Can you work these out from the model? Positions are in its coordinate system, mm. Face numbers are marked on the shaded views. A direction names the side the tool comes from. Give positions to 0.01 mm unless a question says otherwise; leave off trailing zeros. Loops run counter-clockwise (first coordinate to the right, second up) from the corner with the lowest first, then second, coordinate; pieces in that order, holes last. Notation, with made-up numbers: (-7, 82.5) - (39, 82.5) arc R12 cw to (39, 92.5) - close; hole circle Ø5 at (37, 68.25). An arc over 180 degrees is marked (long way). Write item = value, one per line.
from build123d import *

# Parameters (mm, degrees)
F1_DEPTH = 200
F2_T     = -1
F6_D     = 20
F7_D     = 20


# Not quite as in the source:
# - the program builds the solid bodies; features that only make, move or delete a surface that nothing else refers to are left out


with BuildPart() as f1:
    # F0 (on Front) → F1 (new body)
    with BuildSketch(Plane.XZ):
        Polygon((0, 400), (0, 0), (200, 0), (1400, 400), (1600, 400), (1600, 800), (1400, 800), (200, 400), align=None)
    extrude(amount=F1_DEPTH)

    # F2
    f2_openings = [f1.faces().sort_by_distance(p)[0] for p in [
        (100, -100, 400),
        (1500, -100, 800),
        (800, -100, 600),
    ]]
    offset(amount=F2_T, openings=f2_openings, kind=Kind.INTERSECTION)

    # F6 (through all)
    with Locations(Plane.XY.offset(401)):
        with Locations((13, -187), (13, -13)):
            Hole(F6_D / 2)

    # F7 (through all)
    with Locations(Plane.XY.offset(401)):
        with Locations((1587, -13), (1587, -187)):
            Hole(F7_D / 2)


solid = f1.part
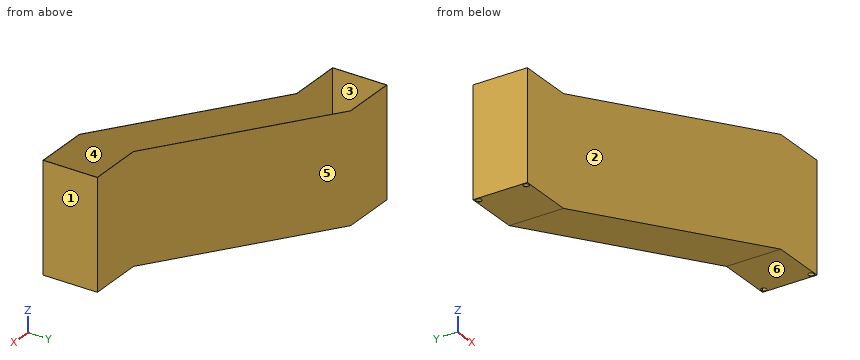
Q1. We'd pull the mould along X, two halves only. Please class the marked faces 1, 2 and 3: released by +X, released by -X, zero draft, split by the parting line, or undercut.
Output:
face_1 = released by +X
face_2 = zero draft
face_3 = undercut
Q2. Imagine slicing it at C-C, the plane y = -40.5. Write out the boundary of the cut face in (x, z), then the cut area to 3 significant figures.
Output:
outline = (0, 0) - (200, 0) - (1400, 400) - (1600, 400) - (1600, 800) - (1599, 800) - (1599, 401) - (1399.84, 401) - (199.84, 1) - (1, 1) - (1, 400) - (0, 400) - close
area = 2,460 mm2
Q3. Imagine slicing it at D-D, the plane z = 106.5. Write out the boundary of the cut face in (x, y).
Output:
outline = (0, -200) - (519.5, -200) - (519.5, 0) - (0, 0) - close; hole (1, -199) - (516.34, -199) - (516.34, -1) - (1, -1) - close
Q4. For pin 1 (1 mm diameter, centred on y = -143.5, z = 495.5, fed in from -X); pin 2 (4 mm diameter, centred on x = 399.5, y = -33.5, fed in from +Z); pin 3 (18 mm diameter, centred on x = 1587, y = -13, fed in from +Z); pin 4 (23 mm diameter, centred on x = 13, y = -187, fed in from +Z), each with a flat end and sliding along its axis, tell me the tip position at first contact or that it passes through.
Output:
pin_1 = 1599
pin_2 = 68.22
pin_3 = through
pin_4 = 1
Q5. I need wall thicknesses on L1, parallel to Y at x = 13, z = 0.6; L2, parallel to Y at x = 348, z = 149; L3, parallel to X at y = -117.5, z = 657. Which ranges of each line are inside material? Lowest first, please.
Output:
L1 = -200 to -197, -177 to -23, -3 to 0
L2 = -200 to -199, -1 to 0
L3 = 1599 to 1600
Q6. Imagine slicing it at A-A, the plane z = 543.5. Write out the boundary of the cut face in (x, y), then the cut area to 3 significant figures.
Output:
outline = (630.5, -200) - (1600, -200) - (1600, 0) - (630.5, 0) - (630.5, -1) - (1599, -1) - (1599, -199) - (630.5, -199) - close
area = 2,140 mm2
Q7. Imagine slicing it at B-B, the plane x = 244.5. Write out the boundary of the cut face in (y, z), then the cut area to 3 significant figures.
Output:
outline = (-200, 14.83) - (0, 14.83) - (0, 414.83) - (-1, 414.83) - (-1, 15.89) - (-199, 15.89) - (-199, 414.83) - (-200, 414.83) - close
area = 1,010 mm2
Q8. Which directions (+Z, -Z, +X, -X, +Y, -Y) give clear straight access to the entire face, cutting with the end or side of a thin tool? Please do the marked faces 4, 5 and 6.
Output:
face_4 = +Z
face_5 = +Z, -Z, +X, -X, +Y
face_6 = -Z, +X, +Y, -Y
